```python
from build123d import *

# Parameters (mm, degrees)
HEX_START         = -3.217333
HEX_2_DEPTH       = 3.217333
CHAMFER1_SIZE     = 0.381
FILLET1_R         = 0.1905
SKETCH3_R         = 2.291358881
HEX_CHAMFER_DEPTH = 2.54
HEX_CHAMFER_DRAFT = 45


with BuildPart() as part:
    # Sketch1 → Body (revolve)
    with BuildSketch(Plane(origin=(0, 0, 0), x_dir=(1, 0, 0), z_dir=(0, 1, 0))):
        Polygon((0, 0), (0, 3.9624), (4.826, 3.9624), (4.826, 2.413), (23.876, 2.413), (23.876, 0), align=None)
    revolve(axis=Axis((23.876, 0, 0), (-1, 0, 0)))

    # Sketch2 → Hex 2 (cut)
    with BuildSketch(Plane.ZY.offset(HEX_START)):
        Polygon((-2.291358881, 0), (-1.14567944, -1.984375), (1.14567944, -1.984375), (2.291358881, 0), (1.14567944, 1.984375), (-1.14567944, 1.984375), align=None)
    extrude(amount=HEX_2_DEPTH, mode=Mode.SUBTRACT)

    # Chamfer1
    chamfer1_edges = [part.edges().sort_by_distance(p)[0] for p in [
        (0, 0, 3.9624),
        (23.876, 0, 2.413),
    ]]
    chamfer(chamfer1_edges, length=CHAMFER1_SIZE)

    # Fillet1
    fillet1_edges = [part.edges().sort_by_distance(p)[0] for p in [
        (4.826, 0, 2.413),
    ]]
    fillet(fillet1_edges, radius=FILLET1_R)


with BuildPart() as hex_chamfer_tool:
    # Sketch3 → Hex Chamfer (with draft: the straight prism first)
    with BuildSketch(Plane(origin=(0, 0, 0), x_dir=(0, 0, -1), z_dir=(1, 0, 0))):
        Circle(SKETCH3_R)
    extrude(amount=HEX_CHAMFER_DEPTH)
    # Hex Chamfer: the draft: its side faces are tilted about the plane it starts from
    hex_chamfer_sides = [hex_chamfer_tool.faces().sort_by_distance(p)[0] for p in [
        (1.27, 0, 2.291358881),
    ]]
    draft(hex_chamfer_sides, Plane(origin=(0, 0, 0), x_dir=(0, 0, -1), z_dir=(1, 0, 0)), HEX_CHAMFER_DRAFT)


with BuildPart() as part_1:
    add(part.part)

    # Hex Chamfer: cut by hex_chamfer_tool
    add(hex_chamfer_tool.part, mode=Mode.SUBTRACT)


solid = part_1.part
```
Can you work these out from the model? Positions are in its coordinate system, mm. A direction names the side the tool comes from. Round coordinates to 2 decimals unless told otherwise and drop trailing zeros. Loops run counter-clockwise (first coordinate to the right, second up) from the corner with the lowest first, then second, coordinate; pieces in that order, holes last.
Item 1: If we mould it in two halves opening along Y, with no side actions, what happens to faces 4 (the flat face through (4.826, 1, -3)), 5 (the cylindrical face through (2.63, -3.93, 0.52)), 6 (the flat face through (1.63, -1.01, 1.71))? For each: +Y half, -Y half, draft (parallel to the pull), parting line (faces both ways), or undercut.
Item 2: Please list where these lines run through material, in increasing order: L1, parallel to X at y = -0.5, z = -3.25; L2, parallel to Z at x = 9.25, y = -0.75; L3, parallel to X at y = 1, z = -1.25.
Item 3: Suppose I cut it at B-B, the plane x = 6.75. Write out the boundary of the cut face in (y, z).
Item 4: Will this pin go through, and if not, where does the flat tip stop? pin 1 Ø3 at (x, y) = (15, 1) entering from +Z.
Item 5: Which directions (+Z, -Z, +X, -X, +Y, -Y) give clear straight access to the entire face, cutting with the end or side of a thin tool? Please do faces 1 (the flat face through (1.631, -0.978, -1.727)), 2 (the cylindrical face through (14.385, 1.468, 1.915)), 3 (the flat face through (0, 0.75, 2.34)).
Reported:
1. face 4: draft
1. face 5: parting line
1. face 6: undercut
2. L1: x = 0 to 4.83
2. L2: z = -2.29 to 2.29
2. L3: x = 3.22 to 23.88
3. outline: circle Ø4.83 at (0, 0)
4. pin 1: stops at z = 2.41
5. face 1: -X
5. face 2: +X
5. face 3: +Z, -Z, -X, +Y, -Y
